```python
from build123d import *

# Parameters (mm, degrees)
BOSS_EXTRUDE1_DEPTH = 13.081
CUT_EXTRUDE1_START  = -11.1252
CUT_EXTRUDE1_DEPTH  = 11.1252
FILLET1_R           = 2.032
FILLET2_R           = 0.762
FILLET6_R           = 1.524
SKETCH6_R           = 3.9751


# Read off the part's stored shape, not the designer's step: Cut-Extrude1
with BuildPart() as part:
    # Sketch1 → Boss-Extrude1 (new, symmetric)
    with BuildSketch(Plane(origin=(0, 0, 0), x_dir=(1, 0, 0), z_dir=(0, 1, 0))):
        Polygon((27.9502, 12.7), (27.9502, 11.1252), (63.561, 11.1252), (63.561, 0), (20, 0), (20, 12.7), align=None)
    extrude(amount=BOSS_EXTRUDE1_DEPTH, both=True)

    # Cut-Extrude1 outline → Cut-Extrude1 (cut)
    with BuildSketch(Plane.XY.offset(CUT_EXTRUDE1_START)):
        Polygon((62.545, 5.5626), (62.545, -5.5626), (46.421739169, -13.081), (63.561, -13.081), (63.561, 13.081), (46.421739169, 13.081), align=None)
    extrude(amount=CUT_EXTRUDE1_DEPTH, mode=Mode.SUBTRACT)

    # Fillet1
    fillet1_edges = [part.edges().sort_by_distance(p)[0] for p in [
        (27.9502, 13.081, -11.9126),
        (46.421739169, -13.081, -5.5626),
        (46.421739169, 13.081, -5.5626),
        (62.545, -5.5626, -5.5626),
        (62.545, 5.5626, -5.5626),
        (20, 13.081, -6.35),
        (27.9502, -13.081, -11.9126),
        (20, -13.081, -6.35),
    ]]
    fillet(fillet1_edges, radius=FILLET1_R)

    # Fillet2
    fillet2_edges = [part.edges().sort_by_distance(p)[0] for p in [
        (23.9751, -13.081, -12.7),
        (23.9751, 13.081, -12.7),
        (27.9502, 0, -12.7),
        (20, 0, -12.7),
        (20.595159021, -12.485840979, -12.7),
        (20.595159021, 12.485840979, -12.7),
        (27.355040979, 12.485840979, -12.7),
        (27.355040979, -12.485840979, -12.7),
    ]]
    fillet(fillet2_edges, radius=FILLET2_R)

    # Fillet6
    fillet6_edges = [part.edges().sort_by_distance(p)[0] for p in [
        (35.944727807, -13.081, -11.1252),
        (34.001627807, -13.081, 0),
        (54.100888115, 9.500154038, 0),
        (34.001627807, 13.081, 0),
        (20, 0, 0),
        (54.100888115, -9.500154038, 0),
        (62.545, 0, 0),
        (62.226771418, 5.359866034, 0),
        (62.226771418, -5.359866034, 0),
        (20.595159021, -12.485840979, 0),
        (20.595159021, 12.485840979, 0),
        (46.41106091, 13.032833486, 0),
        (46.41106091, -13.032833486, 0),
        (54.100888115, -9.500154038, -11.1252),
        (54.100888115, 9.500154038, -11.1252),
        (62.545, 0, -11.1252),
        (35.944727807, 13.081, -11.1252),
        (62.226771418, 5.359866034, -11.1252),
        (62.226771418, -5.359866034, -11.1252),
        (46.41106091, 13.032833486, -11.1252),
        (46.41106091, -13.032833486, -11.1252),
    ]]
    fillet(fillet6_edges, radius=FILLET6_R)

    # Sweep1: sweep along a path in Sketch4
    with BuildLine(Plane(origin=(0, 0, 0), x_dir=(1, 0, 0), z_dir=(0, 1, 0))) as sweep1_path:
        Line((62.545, 5.5626), (81.595, 5.5626))
        ThreePointArc((81.595, 5.5626), (104.045640303, -3.736759697), (113.345, -26.1874))
        Line((113.345, -26.1874), (113.345, -96.0374))
    # Sketch6 → Sweep1 (sweep)
    with BuildSketch(Plane(origin=(62.545, 0, 0), x_dir=(0, 0, -1), z_dir=(1, 0, 0))):
        with Locations((5.5626, 0)):
            Circle(SKETCH6_R)
    sweep(path=sweep1_path.line)


solid = part.part
```
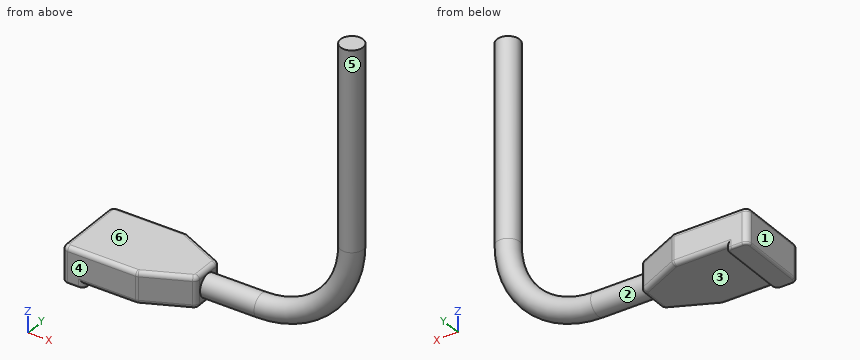
Geometry check sheet. Reference: the model listing, model coordinates, mm. Face numbers are marked on the shaded views. A direction names the side the tool comes from. Give positions to 0.01 mm unless a question says otherwise; leave off trailing zeros. Loops run counter-clockwise (first coordinate to the right, second up) from the corner with the lowest first, then second, coordinate; pieces in that order, holes last. Notation, with made-up numbers: M 9.25,-29 L 22.25,-29 A29 ccw 22.25,-8 Z; hole C 0.25,15.25 d8. An arc over 180 degrees is marked long. Write item = value, one per line.
(1) Material ranges on line 1 (Z direction, x = 29, y = 11.5); line 2 (Y direction, x = 98, z = -4); line 3 (Z direction, x = 113, y = 0.25), recorded low to high. Write a range as [from, to].
Answer below:
line_1 = [-11.13, 0]
line_2 = [-3, 3]
line_3 = [9.17, 96.04]
(2) Tool access check on the marked faces 4, 5 and 6. Record the directions out of +Z, -Z, +X, -X, +Y, -Y that give a thin tool (end or side, any length) a straight path to the whole face; none if there is none.
Answer below:
face_4 = +Z, -Z, +X, -X, -Y
face_5 = +Z
face_6 = +Z, -X, +Y, -Y
(3) Sectioned sample at C-C, the plane z = 89.5. Record the cut outline in (x, y) (3 decimals), plus the area to 3 significant figures.
Answer below:
outline = C 113.345,0 d7.95
area = 49.6 mm2
(4) Sectioned sample at A-A, the plane x = 40. Record the cut outline in (y, z), plus the area to 3 significant figures.
Answer below:
outline = M -13.08,-9.6 A1.52 ccw -11.56,-11.13 L 11.56,-11.13 A1.52 ccw 13.08,-9.6 L 13.08,-1.52 A1.52 ccw 11.56,0 L -11.56,0 A1.52 ccw -13.08,-1.52 Z
area = 289 mm2
(5) Gauge pin test, flat ends, axial feed: pin 1 Ø6 at (y, z) = (-9, 52) entering from -X; pin 2 Ø2 at (x, y) = (42.5, -2.5) entering from +Z; pin 3 Ø3 at (x, y) = (101, 4.5) entering from +Z; pin 4 Ø12 at (y, z) = (-1.5, 58.5) entering from -X. Record the tip position at first contact, or that the pin passes through.
Answer below:
pin_1 = through
pin_2 = 0
pin_3 = 4.8
pin_4 = 109.37
(6) Release check for a two-part mould opening along X. For the marked faces 1, 2 and 3 record: released by +X, released by -X, zero draft, split by the parting line, or undercut.
Answer below:
face_1 = released by -X
face_2 = undercut
face_3 = zero draft
